from build123d import *

# Parameters (mm, degrees)
F0_W     = 6
F0_H     = 7
F1_DEPTH = 8
F2_W     = 3
F2_H     = 7.5
F3_DEPTH = 2
F5_DEPTH = 3


with BuildPart() as f1:
    # F0 (on Front) → F1 (new body)
    with BuildSketch(Plane.XZ):
        with Locations((0, 13.483554)):
            Rectangle(F0_W, F0_H)
    extrude(amount=F1_DEPTH)

    # F2 (on Front) → F3 (cut)
    with BuildSketch(Plane.XZ):
        with Locations((0, 13.472562)):
            Rectangle(F2_W, F2_H)
    extrude(amount=F3_DEPTH, mode=Mode.SUBTRACT)

    # F4 (on Right) → F5 (join, symmetric)
    with BuildSketch(Plane.YZ):
        with BuildLine():
            Line((-7.866293, 10.309412), (-6.651026, 16.728764))
            ThreePointArc((-6.651026, 16.728764), (-14.93047, 16.076312), (-21.348331, 10.805075))
            ThreePointArc((-21.348331, 10.805075), (-14.532663, 12.587694), (-7.866293, 10.309412))
        make_face()
    extrude(amount=F5_DEPTH, both=True)


solid = f1.part
Could you check a few things on this model? Use its own coordinates, in mm. A direction names the side the tool comes from. Coordinates: 2 decimals unless noted, no trailing zeros. Write each loop counter-clockwise with the first axis right and the second up, starting at its lowest first coordinate (ties: lowest second). Pieces come first, ordered by that corner, then holes. Notation, with made-up numbers: M 36.5,83 L 46.5,83 A23 ccw 46.5,110 Z; hole C 46.5,76.5 d7. An arc over 180 degrees is marked long. One line per question, with ' | ' between items.
1) For faces 4 (the face through (-3, -8, 13)), 5 (the face through (-1.5, -1, 13)), which set-ups out of +Z, -Z, +X, -X, +Y, -Y let a thin tool reach every point of the face, with its end or its side?
Checks:
face 4: +Z, -Z, -X, +Y, -Y | face 5: +Z, -Z, +Y
2) I need wall thicknesses on probe 1 along Z at (x, y) = (-0.1, -4.75); probe 2 along Y at (x, z) = (-2.55, 11.25); probe 3 along Z at (x, y) = (-2.75, -9.5). Which ranges of each line are inside material? Lowest first, please. Write a range as [from, to].
Checks:
probe 1: [9.98, 16.98] | probe 2: [-21.05, -20.56], [-9.41, 0] | probe 3: [11.3, 17.08]
3) For pin 1 Ø3 at (x, y) = (-2, -3.5) entering from +Z; pin 2 Ø0.9 at (x, z) = (-0.5, 14.5) entering from +Y; pin 3 Ø1.5 at (x, z) = (2, 14.5) entering from -Y, each with a flat end and sliding along its axis, tell me the tip position at first contact or that it passes through.
Checks:
pin 1: z = 16.98 | pin 2: y = -2 | pin 3: y = -18.76
4) Imagine slicing it at A-A, the plane z = 12.25. Write out the boundary of the cut face in (x, y), and give its area (3 significant figures).
Checks:
outline: M -3,-20.26 L 3,-20.26 L 3,-17.87 L -3,-17.87 Z; M -3,-12.1 L 3,-12.1 L 3,0 L 1.5,0 L 1.5,-2 L -1.5,-2 L -1.5,0 L -3,0 Z | area: 80.9 mm²
5) If we mould it in two halves opening along Y, with no side actions, what happens to faces 1 (the face through (0.042, -14.713, 12.593)), 2 (the face through (0, -4, 16.984)), 3 (the face through (2, 0, 14))? For each: released by +Y, released by -Y, zero draft, split by the parting line, or undercut.
Checks:
face 1: undercut | face 2: zero draft | face 3: released by +Y
6) Imagine slicing it at C-C, the plane z = 13.75. Write out the boundary of the cut face in (x, y), and give its area (3 significant figures).
Checks:
outline: M -3,-18.76 L 3,-18.76 L 3,0 L 1.5,0 L 1.5,-2 L -1.5,-2 L -1.5,0 L -3,0 Z | area: 107 mm²
7) Imagine slicing it at D-D, the plane y = -19.25. Write out the boundary of the cut face in (x, z).
Checks:
outline: M -3,11.83 L 3,11.83 L 3,13.31 L -3,13.31 Z
